```python
from build123d import *

# Parameters (mm, degrees)
SKETCH1_W               = 150
SKETCH1_H               = 200
BOSS_EXTRUDE1_DEPTH     = 50
SHELL1_T                = -3
SKETCH2_W               = 97
SKETCH2_H               = 40.5
CUT_EXTRUDE1_DEPTH      = 40
SKETCH4_R               = 3.5
BOSS_EXTRUDE2_DEPTH     = 6
SKETCH5_R               = 1.5
CUT_EXTRUDE2_DEPTH      = 6
CUT_EXTRUDE3_DEPTH      = 16
CUT_EXTRUDE4_DEPTH      = 185.686220385
CUT_EXTRUDE4_DEPTH_BACK = 185.686220385
SKETCH9_R               = 1.5
SKETCH11_R              = 1.5
SKETCH11_W              = 21
SKETCH11_H              = 16
CUT_EXTRUDE5_DEPTH      = 217.642562762
SKETCH13_R              = 3.5
BOSS_EXTRUDE5_DEPTH     = 6
FILLET1_R               = 7
SKETCH15_R              = 3.5
SKETCH15_R_2            = 1.5
BOSS_EXTRUDE6_DEPTH     = 6
SKETCH17_W              = 66
SKETCH17_H              = 70
BOSS_EXTRUDE7_DEPTH     = 40
SKETCH18_W              = 60
SKETCH18_H              = 34
CUT_EXTRUDE6_DEPTH      = 67
SKETCH19_W              = 30
SKETCH19_H              = 34
CUT_EXTRUDE7_DEPTH      = 3
CHAMFER1_SIZE           = 15
FILLET2_START           = 6
FILLET2_DEPTH           = 3


with BuildPart() as part:
    # Sketch1 → Boss-Extrude1 (new body)
    with BuildSketch(Plane(origin=(0, 0, 0), x_dir=(1, 0, 0), z_dir=(0, 1, 0))):
        Rectangle(SKETCH1_W, SKETCH1_H)
    extrude(amount=BOSS_EXTRUDE1_DEPTH)

    # Shell1
    shell1_openings = [part.faces().sort_by_distance(p)[0] for p in [
        (0, 50, 0),
    ]]
    offset(amount=SHELL1_T, openings=shell1_openings, kind=Kind.INTERSECTION)

    # Sketch2 → Cut-Extrude1 (cut)
    with BuildSketch(Plane(origin=(0, 3, 0), x_dir=(1, 0, 0), z_dir=(0, 1, 0))):
        with Locations((0, 56.75)):
            Rectangle(SKETCH2_W, SKETCH2_H)
    extrude(amount=-CUT_EXTRUDE1_DEPTH, mode=Mode.SUBTRACT)

    # Sketch4 → Boss-Extrude2 (add)
    with BuildSketch(Plane(origin=(0, 3, 0), x_dir=(1, 0, 0), z_dir=(0, 1, 0))):
        with Locations(Location((46.5, 83.7, 0), (0, 0, 90))):
            Circle(SKETCH4_R)
        with Locations(Location((-46.5, 83.7, 0), (0, 0, 90))):
            Circle(SKETCH4_R)
        with Locations(Location((46.5, 29.8, 0), (0, 0, 90))):
            Circle(SKETCH4_R)
        with Locations(Location((-46.5, 29.8, 0), (0, 0, 90))):
            Circle(SKETCH4_R)
    extrude(amount=BOSS_EXTRUDE2_DEPTH)

    # Sketch5 → Cut-Extrude2 (cut)
    with BuildSketch(Plane(origin=(0, 9, 0), x_dir=(1, 0, 0), z_dir=(0, 1, 0))):
        with Locations(Location((-46.5, 83.7, 0), (0, 0, 270))):
            Circle(SKETCH5_R)
        with Locations(Location((46.5, 83.7, 0), (0, 0, 270))):
            Circle(SKETCH5_R)
        with Locations(Location((-46.5, 29.8, 0), (0, 0, 270))):
            Circle(SKETCH5_R)
        with Locations(Location((46.5, 29.8, 0), (0, 0, 270))):
            Circle(SKETCH5_R)
    extrude(amount=-CUT_EXTRUDE2_DEPTH, mode=Mode.SUBTRACT)

    # Sketch7 → Cut-Extrude3 (cut)
    with BuildSketch(Plane(origin=(0, 50, 0), x_dir=(1, 0, 0), z_dir=(0, 1, 0))):
        Polygon((-72, -97), (-72, -80.924133637), (-69, -80.924133637), (-69, -231.933334159), align=None)
        Polygon((69, -231.933334159), (72, -97), (72, -80.924133637), (69, -80.924133637), align=None)
    extrude(amount=-CUT_EXTRUDE3_DEPTH, mode=Mode.SUBTRACT)

    # Sketch9 → Cut-Extrude4 (cut, two sides: drawn at the far end of the back side and taken through both)
    with BuildSketch(Plane(origin=(-72, 0, 0), x_dir=(0, 0, -1), z_dir=(1, 0, 0)).offset(-CUT_EXTRUDE4_DEPTH_BACK)):
        with Locations((-81, 42)):
            Circle(SKETCH9_R)
    extrude(amount=CUT_EXTRUDE4_DEPTH + CUT_EXTRUDE4_DEPTH_BACK, mode=Mode.SUBTRACT)

    # Sketch11 → Cut-Extrude5 (cut, through all)
    with BuildSketch(Plane(origin=(0, 0, 97), x_dir=(-1, 0, 0), z_dir=(0, 0, -1))):
        with Locations((13.5, 26.985710618)):
            Circle(SKETCH11_R)
        with Locations((0, 26.985710618)):
            Rectangle(SKETCH11_W, SKETCH11_H)
    extrude(amount=-CUT_EXTRUDE5_DEPTH, mode=Mode.SUBTRACT)

    # Sketch13 → Boss-Extrude5 (add)
    with BuildSketch(Plane(origin=(0, 50, 0), x_dir=(1, 0, 0), z_dir=(0, 1, 0))):
        with BuildLine():
            Line((-7.5, 106.556339799), (-7.5, 97))
            Line((-7.5, 97), (7.5, 97))
            Line((7.5, 97), (7.5, 106.556339799))
            ThreePointArc((7.5, 106.556339799), (0, 114.056339799), (-7.5, 106.556339799))
        make_face()
        with Locations(Location((0, 106.556339799, 0), (0, 0, 270))):
            Circle(SKETCH13_R, mode=Mode.SUBTRACT)
    extrude(amount=-BOSS_EXTRUDE5_DEPTH)

    # Fillet1
    fillet1_edges = [part.edges().sort_by_distance(p)[0] for p in [
        (0, 3, 97),
    ]]
    fillet(fillet1_edges, radius=FILLET1_R)

    # Sketch15 → Boss-Extrude6 (add)
    # profile 1 of 4: a face of its own
    with BuildSketch(Plane(origin=(0, 3, 0), x_dir=(1, 0, 0), z_dir=(0, 1, 0))):
        with Locations(Location((-58.019508849, -49.793289196, 0), (0, 0, 90))):
            Circle(SKETCH15_R)
        with Locations(Location((-58.019508849, -49.793289196, 0), (0, 0, 270))):
            Circle(SKETCH15_R_2, mode=Mode.SUBTRACT)
    # profile 2 of 4: a face of its own
    with BuildSketch(Plane(origin=(0, 3, 0), x_dir=(1, 0, 0), z_dir=(0, 1, 0))):
        with Locations(Location((-10.019508849, -49.793289196, 0), (0, 0, 90))):
            Circle(SKETCH15_R)
        with Locations(Location((-10.019508849, -49.793289196, 0), (0, 0, 270))):
            Circle(SKETCH15_R_2, mode=Mode.SUBTRACT)
    # profile 3 of 4: a face of its own
    with BuildSketch(Plane(origin=(0, 3, 0), x_dir=(1, 0, 0), z_dir=(0, 1, 0))):
        with Locations(Location((-23.970029682, 0.819287981, 0), (0, 0, 90))):
            Circle(SKETCH15_R)
        with Locations(Location((-23.970029682, 0.819287981, 0), (0, 0, 270))):
            Circle(SKETCH15_R_2, mode=Mode.SUBTRACT)
    # profile 4 of 4: a face of its own
    with BuildSketch(Plane(origin=(0, 3, 0), x_dir=(1, 0, 0), z_dir=(0, 1, 0))):
        with Locations(Location((-51.970029682, 0.819287981, 0), (0, 0, 90))):
            Circle(SKETCH15_R)
        with Locations(Location((-51.970029682, 0.819287981, 0), (0, 0, 270))):
            Circle(SKETCH15_R_2, mode=Mode.SUBTRACT)
    extrude(amount=BOSS_EXTRUDE6_DEPTH)

    # Sketch17 → Boss-Extrude7 (add)
    with BuildSketch(Plane(origin=(0, 3, 0), x_dir=(1, 0, 0), z_dir=(0, 1, 0))):
        with Locations((39, -31.868850241)):
            Rectangle(SKETCH17_W, SKETCH17_H)
    extrude(amount=BOSS_EXTRUDE7_DEPTH)

    # Sketch18 → Cut-Extrude6 (cut)
    with BuildSketch(Plane(origin=(0, 0, -3.131149759), x_dir=(-1, 0, 0), z_dir=(0, 0, -1))):
        with Locations((-39, 23)):
            Rectangle(SKETCH18_W, SKETCH18_H)
    extrude(amount=-CUT_EXTRUDE6_DEPTH, mode=Mode.SUBTRACT)

    # Sketch19 → Cut-Extrude7 (cut)
    with BuildSketch(Plane.ZY.offset(-6)):
        with Locations((44.62857151, 23)):
            Rectangle(SKETCH19_W, SKETCH19_H)
    extrude(amount=-CUT_EXTRUDE7_DEPTH, mode=Mode.SUBTRACT)

    # Chamfer1
    chamfer1_edges = [part.edges().sort_by_distance(p)[0] for p in [
        (7.5, 40, 59.62857151),
        (7.5, 40, 29.62857151),
    ]]
    chamfer(chamfer1_edges, length=CHAMFER1_SIZE - 0.0001)  # a hair under: the kernel refuses the full size


with BuildPart() as fillet2_tool:
    # Fillet2: read off the stored shape, not the designer's step
    # Fillet2 outline → Fillet2 (new body)
    with BuildSketch(Plane.YZ.offset(FILLET2_START)):
        with BuildLine():
            Line((38, 46.62857151), (39.292893219, 45.335678291))
            ThreePointArc((39.292893219, 45.335678291), (39.585786438, 44.628571509), (39.292893219, 43.921464728))
            Line((39.292893219, 43.921464728), (38, 42.628571509))
            Line((38, 42.628571509), (38, 42))
            Line((38, 42), (41, 42))
            Line((41, 42), (41, 47))
            Line((41, 47), (38, 47))
            Line((38, 47), (38, 46.62857151))
        make_face()
    extrude(amount=FILLET2_DEPTH)


with BuildPart() as part_1:
    add(part.part)


with BuildPart() as part_2:
    # Fillet2: joined with fillet2_tool
    add(part_1.part.fuse(fillet2_tool.part, tol=0.00001))


solid = part_2.part
```
Here's how the part is built. I have some questions about the finished solid (model axes, mm). A direction names the side the tool comes from. Give positions to 0.01 mm unless a question says otherwise; leave off trailing zeros. Loops run counter-clockwise (first coordinate to the right, second up) from the corner with the lowest first, then second, coordinate; pieces in that order, holes last. Notation, with made-up numbers: M -14.5,82 L 21.5,82 A29 cw 21.5,112 Z; hole C 58.5,55.5 d9. An arc over 180 degrees is marked long. Put each result on its own line as item: value. Start each with the question number.
(1) I want a section at A-A on x = -33. Please give me the cut outline in (y, z).
(2) For faces 1 (the flat face through (-7.5, 47, -103)), 2 (the flat face through (9, 23, 22)), 3 (the flat face through (-1, 0, -1)), 4 (the flat face through (48, 9, -84.4)), which set-ups out of +Z, -Z, +X, -X, +Y, -Y let a thin tool reach every point of the face, with its end or its side?
(3) I want a section at B-B on z = 25.5. Please give me the cut outline in (x, y), then the cut area to 3 significant figures.
(4) If we mould it in two halves opening along Z, with no side actions, what happens to faces 5 (the flat face through (7.5, 47, -103)), 6 (the cylindrical face through (43.55, 5.96, -85.58))? For each: +Z half, -Z half, draft (parallel to the pull), parting line (faces both ways), or undercut.
(5) I want a section at D-D on z = -21.5. Please give me the cut outline in (x, y).
(6) I want a section at C-C on x = 53.5. Please give me the cut outline in (y, z), then the cut area to 3 significant figures.
(7) Will these pins go through, and if not, where does the flat tip stop? pin 1 Ø2 at (x, z) = (-53.5, 0.5) entering from +Y; pin 2 Ø5 at (x, z) = (-35, 27.5) entering from +Y; pin 3 Ø8 at (x, y) = (58.5, 32.5) entering from -Z.
(8) I need wall thicknesses on line 1 along Z through (x, y) = (58, 11.5); line 2 along X through (y, z) = (28, 30.5); line 3 along X through (y, z) = (4.55, -83.7). Which ranges of each line are inside material? Lowest first, please. Write a range as [from, to].
Answer block:
1. outline: M 0,-100 L 50,-100 L 50,-97 L 3,-97 L 3,-77 L 0,-77 Z; M 0,-36.5 L 3,-36.5 L 3,90 A7 cw 10,97 L 50,97 L 50,100 L 0,100 Z
2. face 1: -Z, -X, +Y, -Y
2. face 2: none
2. face 3: +Z, -Z, +X, -X, -Y
2. face 4: +Y
3. outline: M -75,0 L 75,0 L 75,50 L 72,50 L 72,43 L 6,43 L 6,3 L -72,3 L -72,50 L -75,50 Z; hole M 9,6 L 69,6 L 69,40 L 9,40 Z
3. area: 1,330 mm^2
4. face 5: draft
4. face 6: undercut
5. outline: M -75,0 L 75,0 L 75,50 L 72,50 L 72,3 L -72,3 L -72,50 L -75,50 Z
6. outline: M 0,-100 L 50,-100 L 50,-97 L 3,-97 L 3,-3.13 L 6,-3.13 L 6,63.87 L 40,63.87 L 40,-3.13 L 43,-3.13 L 43,66.87 L 3,66.87 L 3,90 A7 cw 10,97 L 50,97 L 50,100 L 0,100 Z
6. area: 1,410 mm^2
7. pin 1: y = 9
7. pin 2: y = 3
7. pin 3: z = -100
8. line 1: [-100, -97], [63.87, 66.87], [97, 100]
8. line 2: [-75, -72], [6, 9], [69, 75]
8. line 3: [-75, -72], [-50, -48], [-45, -43], [43, 45], [48, 50], [72, 75]
